Here's how the part is built. I have some questions about the finished solid (model axes, mm). Round coordinates to 2 decimals unless told otherwise and drop trailing zeros. Order: outer loops, then holes, each group sorted by start corner. A loop starts at its lowest first (then second) coordinate and runs counter-clockwise, first axis right, second up. Notation, with made-up numbers: M 66,83.5 L 114,83.5 A22 ccw 114,113.5 Z; hole C 15,71 d5. An arc over 180 degrees is marked long. Use one line per item in the form item = value. Start each with the question number.
```python
from build123d import *

# Parameters (mm, degrees)
SKETCH1_W           = 226
SKETCH1_H           = 198
BOSS_EXTRUDE1_DEPTH = 3
INPUT_FOR_SPEAKER_R = 5
CUT_EXTRUDE1_DEPTH  = 10
FILLET1_R           = 10


with BuildPart() as part:
    # Sketch1 → Boss-Extrude1 (new body)
    with BuildSketch(Plane(origin=(0, 0, 0), x_dir=(1, 0, 0), z_dir=(0, 1, 0))):
        with Locations((113, 99)):
            Rectangle(SKETCH1_W, SKETCH1_H)
    extrude(amount=BOSS_EXTRUDE1_DEPTH)

    # Input for speaker → Cut-Extrude1 (cut)
    with BuildSketch(Plane(origin=(0, 3, 0), x_dir=(1, 0, 0), z_dir=(0, 1, 0))):
        with Locations(Location((113, 99.5, 0), (0, 0, 270))):
            Circle(INPUT_FOR_SPEAKER_R)
    extrude(amount=-CUT_EXTRUDE1_DEPTH, mode=Mode.SUBTRACT)

    # Fillet1
    fillet1_edges = [part.edges().sort_by_distance(p)[0] for p in [
        (226, 1.5, 0),
        (0, 1.5, 0),
    ]]
    fillet(fillet1_edges, radius=FILLET1_R)


solid = part.part
```
1) If we mould it in two halves opening along X, with no side actions, what happens to faces 1 (the cylindrical face through (2.85, 1.52, -3.01)), 2 (the flat face through (111, 0, -122)), 3 (the cylindrical face through (222.99, 1.52, -2.85)), 4 (the cylindrical face through (111.085, 1.521, -94.881))? For each: +X half, -X half, draft (parallel to the pull), parting line (faces both ways), or undercut.
2) If I drill on line 1 (X direction, y = 2.15, z = -99.5), over which ranges is the centre line in solid material (lowest first)?
3) If we section it at A-A on x = 113: Write out the boundary of the cut face in (y, z).
4) If we section it at B-B on z = -99.5: Write out the boundary of the cut face in (x, y), then the cut area to 3 significant figures.
Completed:
q1.face_1 = -X half
q1.face_2 = draft
q1.face_3 = +X half
q1.face_4 = undercut
q2.line_1 = 0 to 108, 118 to 226
q3.outline = M 0,-198 L 3,-198 L 3,-104.5 L 0,-104.5 Z; M 0,-94.5 L 3,-94.5 L 3,0 L 0,0 Z
q4.outline = M 0,0 L 108,0 L 108,3 L 0,3 Z; M 118,0 L 226,0 L 226,3 L 118,3 Z
q4.area = 648 mm²
